```python
from build123d import *

# Parameters (mm, degrees)
CUT_EXTRUDE1_START = 1.245
CUT_EXTRUDE1_DEPTH = 7.37
CIRPATTERN1_COUNT  = 12


with BuildPart() as part:
    # Sketch2 → Revolve1 (revolve)
    with BuildSketch(Plane(origin=(0, 0, 0), x_dir=(0, 0, -1), z_dir=(1, 0, 0)), mode=Mode.PRIVATE) as revolve1_sk:
        Polygon((-7.135, 1.5875), (7.135, 1.5875), (7.135, 6.096), (6.63, 6.096), (6.125, 4.83225), (6.125, 3.5685), (-1.245, 3.5685), (-1.245, 4.83225), (-1.75, 6.096), (-7.135, 6.096), align=None)
    revolve(revolve1_sk.sketch.rotate(Axis((0, 0, 7.135), (0, 0, -1)), 90), axis=Axis((0, 0, 7.135), (0, 0, -1)))

    # Sketch3 → Cut-Extrude1 (cut)
    with BuildSketch(Plane.XY.offset(CUT_EXTRUDE1_START)):
        with BuildLine():
            Line((3.566654882, 6.096), (-3.566654882, 6.096))
            Line((-3.566654882, 6.096), (-1.802078902, 3.080049331))
            ThreePointArc((-1.802078902, 3.080049331), (-1.296607682, 3.324605355), (-0.759031417, 3.486841487))
            ThreePointArc((-0.759031417, 3.486841487), (-0.645131247, 3.465879975), (-0.580109509, 3.370042573))
            ThreePointArc((-0.580109509, 3.370042573), (-0.547109503, 3.247589437), (-0.498876404, 3.130297753))
            ThreePointArc((-0.498876404, 3.130297753), (0, 2.8185), (0.498876404, 3.130297753))
            ThreePointArc((0.498876404, 3.130297753), (0.547109503, 3.247589437), (0.580109509, 3.370042573))
            ThreePointArc((0.580109509, 3.370042573), (0.645131247, 3.465879975), (0.759031417, 3.486841487))
            ThreePointArc((0.759031417, 3.486841487), (1.296607682, 3.324605355), (1.802078902, 3.080049331))
            Line((1.802078902, 3.080049331), (3.566654882, 6.096))
        make_face()
    cut_extrude1 = extrude(amount=-CUT_EXTRUDE1_DEPTH, mode=Mode.SUBTRACT)

    # CirPattern1: Cut-Extrude1 ×12 about axis
    cirpattern1_axis = Axis((0, 0, 0), (0, 0, 1))
    for i in range(1, CIRPATTERN1_COUNT):
        add(cut_extrude1.rotate(cirpattern1_axis, i * 360 / CIRPATTERN1_COUNT), mode=Mode.SUBTRACT)


solid = part.part
```
Check sheet for the modelled part. Datum: model origin and axes. Units: mm. A direction names the side the tool comes from. Give positions to 0.01 mm unless a question says otherwise; leave off trailing zeros. Loops run counter-clockwise (first coordinate to the right, second up) from the corner with the lowest first, then second, coordinate; pieces in that order, holes last. Notation, with made-up numbers: M 85.25,28 L 95.25,28 A19 cw 95.25,60 Z; hole C -37.75,-15 d1. An arc over 180 degrees is marked long. Answer as CSV lines item,"result".
Item 1: Draft check along Z on faces 1 (the face through (-1.3, 1.3, -7.135)), 2 (the face through (-1.26, 0.966, -0.1)), 3 (the face through (2.445, -1.402, -2.388)), 4 (the face through (2.437, 1.417, -2.388)). Enter one of: pulls with the +Z half, pulls with the -Z half, needs draft (parallel to the pull), parting line crosses it, or undercut.
Reply:
face 1,"pulls with the -Z half"
face 2,"needs draft"
face 3,"undercut"
face 4,"undercut"
Item 2: Set-up check for faces 5 (the face through (2.82, 0.01, -2.39)), 6 (the face through (-1.402, -2.445, -2.388)), 7 (the face through (0.01, -2.82, -2.39)), 8 (the face through (-0.01, 2.82, -2.39)), 9 (the face through (-2.82, -0.01, -2.39)): record each of +Z, -Z, +X, -X, +Y, -Y from which the full face is reachable in a straight line by a thin tool's end or side.
Reply:
face 5,"+X"
face 6,"none"
face 7,"-Y"
face 8,"+Y"
face 9,"-X"
Item 3: Sectioned sample at C-C, the plane z = 3. Enter the section's corners in (x, y) (1 decimal), then the cut area to 3 significant figures.
Reply:
outline,"C 0,0 d12.2; hole C 0,0 d3.2"
area,"109 mm^2"
Item 4: Scan lines: L1, parallel to Y at x = 0, z = 0; L2, parallel to Z at x = 2.5, y = 1.75 (3 decimals); L3, parallel to Z at x = 1.5, y = -5.5 (3 decimals). Record each from-to range of solid material in increasing order.
Reply:
L1,"-2.82 to -1.59, 1.59 to 2.82"
L2,"-7.135 to -6.125, 1.245 to 7.135"
L3,"-7.135 to -6.472, 1.592 to 7.135"
Item 5: Depth check by flat-ended pin: pin 1 Ø1.5 at (x, z) = (2.5, 4) entering from -Y; pin 2 Ø1.9 at (x, y) = (0, 0) entering from +Z; pin 3 Ø6 at (x, z) = (4.5, -3) entering from +Y; pin 4 Ø1.5 at (y, z) = (2.5, -2) entering from -X. Enter the tip coordinate at first touch or a pass-through.
Reply:
pin 1,"y = -5.84"
pin 2,"through"
pin 3,"y = 2.68"
pin 4,"x = -2.68"
